CAD build for the part. Positions are in the model's coordinates, mm. Face numbers are marked on the shaded views. A direction names the side the tool comes from. Give positions to 0.01 mm unless a question says otherwise; leave off trailing zeros. Write each loop counter-clockwise with the first axis right and the second up, starting at its lowest first coordinate (ties: lowest second). Pieces come first, ordered by that corner, then holes. Notation, with made-up numbers: (74, 38.5) - (93, 38.5) arc R12 ccw to (93, 43.5) - close; hole circle Ø10 at (-27.75, -13). An arc over 180 degrees is marked (long way). Answer as a JSON object with one key per item and string values.
from build123d import *

# Parameters (mm, degrees)
F0_W        = 10
F0_H        = 20
F1_DEPTH    = 25
F3_W        = 30
F3_H        = 20
F4_DEPTH    = 10
F5_T1_DEPTH = 114.1408313715
F6_W        = 11
F6_H        = 20
F7_DEPTH    = 1
F8_W        = 1.1
F8_H        = 3.4004326878
F9_DEPTH    = 5.0529


# Not quite as in the source:
# - a fillet or chamfer that OpenCascade refuses, or shapes differently, is made with other operations: its cross-section is extruded or revolved along the edge and cut away or added


with BuildPart() as f1:
    # F0 (on Front) → F1 (new body)
    with BuildSketch(Plane.XZ):
        Rectangle(F0_W, F0_H)
    extrude(amount=-F1_DEPTH)

    # F3 (on face) → F4 (join)
    with BuildSketch(Plane(origin=(-5, 0, 0), x_dir=(0, -1, 0), z_dir=(-1, 0, 0))):
        with Locations((-39.8661582013, 0)):
            Rectangle(F3_W, F3_H)
    extrude(amount=-F4_DEPTH)

    # F5: fillet of radius 22.7249922626 on 1 edges, made by hand

    # F5_s2 → F5_t1 (cut)
    with BuildSketch(Plane.XY.offset(-57.0704156857)):
        with BuildLine():
            ThreePointArc((-5, 54.8661582013), (2.3448934377, 46.697492915), (5, 36.037991927))
            Line((5, 36.037991927), (5, 54.8661582013))
            Line((5, 54.8661582013), (-5, 54.8661582013))
        make_face()
    extrude(amount=F5_T1_DEPTH, mode=Mode.SUBTRACT)

    # F6 (on face) → F7 (join)
    with BuildSketch(Plane(origin=(-5, 0, 0), x_dir=(0, -1, 0), z_dir=(-1, 0, 0))):
        with Locations((-49.3244222254, 0.0391426826)):
            Rectangle(F6_W, F6_H)
    extrude(amount=F7_DEPTH)

    # F8 (on face) → F9 (join)
    with BuildSketch(Plane.XZ):
        with Locations((-4.05, 7.9997836561)):
            Rectangle(F8_W, F8_H)
        with Locations((-1.35, 7.9997836561)):
            Rectangle(F8_W, F8_H)
        with Locations((1.35, 7.9997836561)):
            Rectangle(F8_W, F8_H)
        with Locations((4.05, 7.9997836561)):
            Rectangle(F8_W, F8_H)
        with Locations((-4.1088341387, 0)):
            Rectangle(F8_W, F8_H)
        with Locations((-4.1676682773, -7.9997836561)):
            Rectangle(F8_W, F8_H)
        with Locations((-1.4088339935, 1.97401e-05)):
            Rectangle(F8_W, F8_H)
        with Locations((-1.467667987, -7.9997441759)):
            Rectangle(F8_W, F8_H)
        with Locations((1.2911689242, 0.0004164637)):
            Rectangle(F8_W, F8_H)
        with Locations((1.2323378484, -7.9989507287)):
            Rectangle(F8_W, F8_H)
        with Locations((3.9911658613, 0)):
            Rectangle(F8_W, F8_H)
        with Locations((3.9323317227, -7.9997836561)):
            Rectangle(F8_W, F8_H)
    extrude(amount=F9_DEPTH)


solid = f1.part
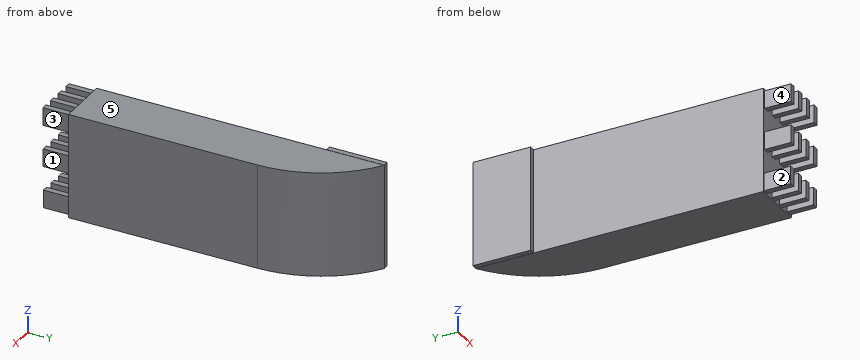
(1) Saw through at D-D, the plane y = 14. Give the cut face in (x, z).
Answer key:
{"outline": "(-5, -10) - (5, -10) - (5, 10) - (-5, 10) - close"}
(2) Flat gauge pins, fed straight in: P1, Ø10, axis at y = 46, z = -2.5, coming from the +X side; P2, Ø0.9, axis at x = -4, y = -3, coming from the -Z side; P3, Ø6, axis at x = -3.5, y = 1, coming from the +Z side. Where does each tip first touch, or does it go through?
Answer key:
{"P1": "stops at x = 4.45", "P2": "stops at z = -9.7", "P3": "stops at z = 10"}
(3) Saw through at C-C, the plane z = 7. Give the cut face in (x, y) (3 decimals).
Answer key:
{"outline": "(-6, 43.824) - (-5, 43.824) - (-5, 0) - (-4.6, 0) - (-4.6, -5.053) - (-3.5, -5.053) - (-3.5, 0) - (-1.9, 0) - (-1.9, -5.053) - (-0.8, -5.053) - (-0.8, 0) - (0.8, 0) - (0.8, -5.053) - (1.9, -5.053) - (1.9, 0) - (3.5, 0) - (3.5, -5.053) - (4.6, -5.053) - (4.6, 0) - (5, 0) - (5, 36.038) arc R22.725 ccw to (-5, 54.866) - (-5, 54.824) - (-6, 54.824) - close"}
(4) Saw through at A-A, the plane z = -4. Give the cut face in (x, y) (3 decimals), and give its area (3 significant figures).
Answer key:
{"outline": "(-6, 43.824) - (-5, 43.824) - (-5, 0) - (5, 0) - (5, 36.038) arc R22.725 ccw to (-5, 54.866) - (-5, 54.824) - (-6, 54.824) - close", "area": "504 mm²"}
(5) 3-axis set-ups, long thin cutter, end or side, ignore diameter. For the marked faces 1, 2, 3, 4 and 5: which of +Z, -Z, +X, -X, +Y, -Y reach the whole face in a straight line?
Answer key:
{"face 1": "-Z, +X, -Y", "face 2": "+Z, -Z, -X, -Y", "face 3": "+Z, -Z, +X, -Y", "face 4": "+Z, -X, -Y", "face 5": "+Z, +X, +Y, -Y"}
(6) Probe L1, parallel to X at y = -1, z = 9; L2, parallel to Z at x = -4, y = 40.5; L3, parallel to X at y = 15, z = -5. List the from-to ranges inside material, lowest first. Write a range as [from, to].
Answer key:
{"L1": "x = [-4.6, -3.5], [-1.9, -0.8], [0.8, 1.9], [3.5, 4.6]", "L2": "z = [-10, 10]", "L3": "x = [-5, 5]"}
